```python
from build123d import *

# Parameters (mm, degrees)
F0_W     = 45
F0_H     = 35
F0_R     = 2.2182693531
F1_DEPTH = 3.5


with BuildPart() as f1:
    # F0 (on Top) → F1 (new body)
    with BuildSketch(Plane.XY):
        with Locations((-22.5, 17.5)):
            Rectangle(F0_W, F0_H)
        with BuildLine():
            Line((-39.1418465407, 16.9395460091), (-37.3351271333, 16.9395460091))
            Line((-37.3351271333, 16.9395460091), (-37.3351271333, 11.41090981))
            add(Edge.make_bspline(
                [(-37.3351271333, 11.41090981), (-37.3351271333, 10.4626626676), (-37.7587523359, 9.7500745783)],
                knots=[0, 0, 0, 1, 1, 1], degree=2))
            add(Edge.make_bspline(
                [(-37.7587523359, 9.7500745783), (-38.1823775386, 9.0374864891), (-38.9838053503, 8.6568784152)],
                knots=[0, 0, 0, 1, 1, 1], degree=2))
            add(Edge.make_bspline(
                [(-38.9838053503, 8.6568784152), (-39.785233162, 8.2762703412), (-40.8774941702, 8.2762703412)],
                knots=[0, 0, 0, 1, 1, 1], degree=2))
            add(Edge.make_bspline(
                [(-40.8774941702, 8.2762703412), (-42.5252372322, 8.2762703412), (-43.4370133307, 9.1216504366)],
                knots=[0, 0, 0, 1, 1, 1], degree=2))
            add(Edge.make_bspline(
                [(-43.4370133307, 9.1216504366), (-44.3487894291, 9.967030532), (-44.3487894291, 11.4333535293)],
                knots=[0, 0, 0, 1, 1, 1], degree=2))
            Line((-44.3487894291, 11.4333535293), (-44.3487894291, 16.9395460091))
            Line((-44.3487894291, 16.9395460091), (-42.5439403317, 16.9395460091))
            Line((-42.5439403317, 16.9395460091), (-42.5439403317, 11.7082890913))
            add(Edge.make_bspline(
                [(-42.5439403317, 11.7082890913), (-42.5439403317, 10.7207654401), (-42.1464994682, 10.2587988835)],
                knots=[0, 0, 0, 1, 1, 1], degree=2))
            add(Edge.make_bspline(
                [(-42.1464994682, 10.2587988835), (-41.7490586048, 9.796832327), (-40.8307364215, 9.796832327)],
                knots=[0, 0, 0, 1, 1, 1], degree=2))
            add(Edge.make_bspline(
                [(-40.8307364215, 9.796832327), (-39.9423391974, 9.796832327), (-39.542092869, 10.2616043485)],
                knots=[0, 0, 0, 1, 1, 1], degree=2))
            add(Edge.make_bspline(
                [(-39.542092869, 10.2616043485), (-39.1418465407, 10.7263763699), (-39.1418465407, 11.719510951)],
                knots=[0, 0, 0, 1, 1, 1], degree=2))
            Line((-39.1418465407, 11.719510951), (-39.1418465407, 16.9395460091))
        make_face(mode=Mode.SUBTRACT)
        with BuildLine():
            add(Edge.make_bspline(
                [(-30.6599909376, 15.3843832893), (-31.1444012135, 15.5536463394), (-31.6119786999, 15.5536463394)],
                knots=[0, 0, 0, 1, 1, 1], degree=2))
            add(Edge.make_bspline(
                [(-31.6119786999, 15.5536463394), (-32.6350382401, 15.5536463394), (-33.1961312237, 14.7849489518)],
                knots=[0, 0, 0, 1, 1, 1], degree=2))
            add(Edge.make_bspline(
                [(-33.1961312237, 14.7849489518), (-33.7572242074, 14.0162515642), (-33.7572242074, 12.6434440641)],
                knots=[0, 0, 0, 1, 1, 1], degree=2))
            add(Edge.make_bspline(
                [(-33.7572242074, 12.6434440641), (-33.7572242074, 9.7856104673), (-31.6119786999, 9.7856104673)],
                knots=[0, 0, 0, 1, 1, 1], degree=2))
            add(Edge.make_bspline(
                [(-31.6119786999, 9.7856104673), (-30.712359616, 9.7856104673), (-29.4330676133, 10.2344848542)],
                knots=[0, 0, 0, 1, 1, 1], degree=2))
            Line((-29.4330676133, 10.2344848542), (-29.4330676133, 8.7157931784))
            add(Edge.make_bspline(
                [(-29.4330676133, 8.7157931784), (-30.4841818027, 8.2762703412), (-31.7821769049, 8.2762703412)],
                knots=[0, 0, 0, 1, 1, 1], degree=2))
            add(Edge.make_bspline(
                [(-31.7821769049, 8.2762703412), (-33.6468759206, 8.2762703412), (-34.6343995719, 9.4078078583)],
                knots=[0, 0, 0, 1, 1, 1], degree=2))
            add(Edge.make_bspline(
                [(-34.6343995719, 9.4078078583), (-35.6219232231, 10.5393453754), (-35.6219232231, 12.6546659238)],
                knots=[0, 0, 0, 1, 1, 1], degree=2))
            add(Edge.make_bspline(
                [(-35.6219232231, 12.6546659238), (-35.6219232231, 13.988196915), (-35.1365777923, 14.9906830458)],
                knots=[0, 0, 0, 1, 1, 1], degree=2))
            add(Edge.make_bspline(
                [(-35.1365777923, 14.9906830458), (-34.6512323614, 15.9931691766), (-33.7422617278, 16.5271426661)],
                knots=[0, 0, 0, 1, 1, 1], degree=2))
            add(Edge.make_bspline(
                [(-33.7422617278, 16.5271426661), (-32.8332910943, 17.0611161555), (-31.6119786999, 17.0611161555)],
                knots=[0, 0, 0, 1, 1, 1], degree=2))
            add(Edge.make_bspline(
                [(-31.6119786999, 17.0611161555), (-30.3682225861, 17.0611161555), (-29.1113743026, 16.460746663)],
                knots=[0, 0, 0, 1, 1, 1], degree=2))
            Line((-29.1113743026, 16.460746663), (-29.6949110057, 14.9869424259))
            add(Edge.make_bspline(
                [(-29.6949110057, 14.9869424259), (-30.1755806617, 15.2151202393), (-30.6599909376, 15.3843832893)],
                knots=[0, 0, 0, 1, 1, 1], degree=2))
        make_face(mode=Mode.SUBTRACT)
        with BuildLine():
            add(Edge.make_bspline(
                [(-20.9025839516, 15.9398653432), (-19.858951002, 14.8055223612), (-19.858951002, 12.6789799531)],
                knots=[0, 0, 0, 1, 1, 1], degree=2))
            add(Edge.make_bspline(
                [(-19.858951002, 12.6789799531), (-19.858951002, 10.5561781649), (-20.9110003463, 9.4162242531)],
                knots=[0, 0, 0, 1, 1, 1], degree=2))
            add(Edge.make_bspline(
                [(-20.9110003463, 9.4162242531), (-21.9630496907, 8.2762703412), (-23.9268751335, 8.2762703412)],
                knots=[0, 0, 0, 1, 1, 1], degree=2))
            add(Edge.make_bspline(
                [(-23.9268751335, 8.2762703412), (-25.8907005764, 8.2762703412), (-26.9427499208, 9.4162242531)],
                knots=[0, 0, 0, 1, 1, 1], degree=2))
            add(Edge.make_bspline(
                [(-26.9427499208, 9.4162242531), (-27.9947992651, 10.5561781649), (-27.9947992651, 12.6902018128)],
                knots=[0, 0, 0, 1, 1, 1], degree=2))
            add(Edge.make_bspline(
                [(-27.9947992651, 12.6902018128), (-27.9947992651, 14.8242254606), (-26.9399444558, 15.9492168929)],
                knots=[0, 0, 0, 1, 1, 1], degree=2))
            add(Edge.make_bspline(
                [(-26.9399444558, 15.9492168929), (-25.8850896466, 17.0742083252), (-23.9156532739, 17.0742083252)],
                knots=[0, 0, 0, 1, 1, 1], degree=2))
            add(Edge.make_bspline(
                [(-23.9156532739, 17.0742083252), (-21.9462169012, 17.0742083252), (-20.9025839516, 15.9398653432)],
                knots=[0, 0, 0, 1, 1, 1], degree=2))
        make_face(mode=Mode.SUBTRACT)
        with BuildLine():
            Line((-10.5074012742, 16.9395460091), (-10.5074012742, 8.3940998678))
            Line((-10.5074012742, 8.3940998678), (-12.8097528171, 8.3940998678))
            Line((-12.8097528171, 8.3940998678), (-16.5279289889, 14.8578910397))
            Line((-16.5279289889, 14.8578910397), (-16.5802976674, 14.8578910397))
            add(Edge.make_bspline(
                [(-16.5802976674, 14.8578910397), (-16.4680790707, 13.1465574395), (-16.4680790707, 12.4152662508)],
                knots=[0, 0, 0, 1, 1, 1], degree=2))
            Line((-16.4680790707, 12.4152662508), (-16.4680790707, 8.3940998678))
            Line((-16.4680790707, 8.3940998678), (-18.0877674835, 8.3940998678))
            Line((-18.0877674835, 8.3940998678), (-18.0877674835, 16.9395460091))
            Line((-18.0877674835, 16.9395460091), (-15.80224873, 16.9395460091))
            Line((-15.80224873, 16.9395460091), (-12.091553798, 10.5393453754))
            Line((-12.091553798, 10.5393453754), (-12.0504069792, 10.5393453754))
            add(Edge.make_bspline(
                [(-12.0504069792, 10.5393453754), (-12.1383115467, 12.2057915369), (-12.1383115467, 12.8940655968)],
                knots=[0, 0, 0, 1, 1, 1], degree=2))
            Line((-12.1383115467, 12.8940655968), (-12.1383115467, 16.9395460091))
            Line((-12.1383115467, 16.9395460091), (-10.5074012742, 16.9395460091))
        make_face(mode=Mode.SUBTRACT)
        with BuildLine():
            Line((-0.7761786274, 16.9395460091), (-0.7761786274, 8.3940998678))
            Line((-0.7761786274, 8.3940998678), (-3.0785301704, 8.3940998678))
            Line((-3.0785301704, 8.3940998678), (-6.7967063422, 14.8578910397))
            Line((-6.7967063422, 14.8578910397), (-6.8490750206, 14.8578910397))
            add(Edge.make_bspline(
                [(-6.8490750206, 14.8578910397), (-6.7368564239, 13.1465574395), (-6.7368564239, 12.4152662508)],
                knots=[0, 0, 0, 1, 1, 1], degree=2))
            Line((-6.7368564239, 12.4152662508), (-6.7368564239, 8.3940998678))
            Line((-6.7368564239, 8.3940998678), (-8.3565448368, 8.3940998678))
            Line((-8.3565448368, 8.3940998678), (-8.3565448368, 16.9395460091))
            Line((-8.3565448368, 16.9395460091), (-6.0710260833, 16.9395460091))
            Line((-6.0710260833, 16.9395460091), (-2.3603311513, 10.5393453754))
            Line((-2.3603311513, 10.5393453754), (-2.3191843325, 10.5393453754))
            add(Edge.make_bspline(
                [(-2.3191843325, 10.5393453754), (-2.4070888999, 12.2057915369), (-2.4070888999, 12.8940655968)],
                knots=[0, 0, 0, 1, 1, 1], degree=2))
            Line((-2.4070888999, 12.8940655968), (-2.4070888999, 16.9395460091))
            Line((-2.4070888999, 16.9395460091), (-0.7761786274, 16.9395460091))
        make_face(mode=Mode.SUBTRACT)
        with Locations((-24.1070296615, 30.3892251104)):
            Circle(F0_R, mode=Mode.SUBTRACT)
    extrude(amount=F1_DEPTH)


solid = f1.part
```
Part model, mm, in its own coordinate system. Round coordinates to 2 decimals unless told otherwise and drop trailing zeros. Write each loop counter-clockwise with the first axis right and the second up, starting at its lowest first coordinate (ties: lowest second). Pieces come first, ordered by that corner, then holes.
Item 1: Drop a flat-ended pin along its axis: pin 1 Ø3.5 at (x, y) = (-24.11, 30.39) entering from -Z. Give the stop position or say it passes through.
Results:
pin 1: passes through
Item 2: Probe L1, parallel to Y at x = -31.5, z = 1.9; L2, parallel to Y at x = -41, z = 1.75; L3, parallel to Y at x = -38, z = 2.45. List the from-to ranges inside material, lowest first.
Results:
L1: y = 0 to 8.28, 9.79 to 15.55, 17.06 to 35
L2: y = 0 to 8.28, 9.8 to 35
L3: y = 0 to 9.41, 16.94 to 35
Item 3: Two-plate mould, pull along X, no slides. Class faces 1 (the flat face through (-23, 18, 3.5)), 2 (the flat face through (-8.357, 13, 2)): +X half, -X half, draft (parallel to the pull), parting line (faces both ways), or undercut.
Results:
face 1: draft
face 2: undercut
Item 4: Cut at A-A, the plane x = -5. Give the cut face in (y, z).
Results:
outline: (0, 0) - (11.73, 0) - (11.73, 3.5) - (0, 3.5) - close; (15.09, 0) - (35, 0) - (35, 3.5) - (15.09, 3.5) - close
Item 5: Cut at B-B, the plane x = -22.5. Count the separate pieces of the cut face and the enclosed holes in it, plus the area to 3 significant figures.
Results:
separate pieces: 3
enclosed holes: 0
area: 82.3 mm2
